```python
from build123d import *

# Parameters (mm, degrees)
F0_R     = 8
F0_R_2   = 16
F1_DEPTH = 19
F0_R_3   = 11
F0_R_4   = 24
F2_DEPTH = 25
F7_DEPTH = 25.001


with BuildPart() as f1:
    # F0 (on Right) → F1 (new body)
    with BuildSketch(Plane.YZ):
        Circle(F0_R)
        Circle(F0_R_2)
        Circle(F0_R, mode=Mode.SUBTRACT)
    extrude(amount=F1_DEPTH)



with BuildPart() as f2:
    # F0 (on Right) → F2 (new body)
    with BuildSketch(Plane.YZ):
        with Locations((0, 140)):
            Circle(F0_R_3)
        with Locations((0, 140)):
            Circle(F0_R_4)
        with Locations((0, 140)):
            Circle(F0_R_3, mode=Mode.SUBTRACT)
    extrude(amount=F2_DEPTH)


with BuildPart() as f1_1:
    add(f1.part)

    add(f2.part)  # F6 merges F2
    # F5 (on plane+point) → F6 section 0
    with BuildSketch(Plane.XY.offset(140)):
        with BuildLine():
            add(Edge.make_bspline(
                [(9, 24), (-1.392305, 24), (3.803848, -12), (9, -48), (14.196152, -12), (19.392305, 24), (9, 24)],
                knots=[0, 0, 0, 2.094395, 2.094395, 4.18879, 4.18879, 6.283185, 6.283185, 6.283185], degree=2, weights=[1, 0.5, 1, 0.5, 1, 0.5, 1]))
        make_face()
    # F3 (on Top) → F6 section 1
    with BuildSketch(Plane.XY):
        with BuildLine():
            add(Edge.make_bspline(
                [(9, 24), (-1.392305, 24), (3.803848, -12), (9, -48), (14.196152, -12), (19.392305, 24), (9, 24)],
                knots=[0, 0, 0, 2.094395, 2.094395, 4.18879, 4.18879, 6.283185, 6.283185, 6.283185], degree=2, weights=[1, 0.5, 1, 0.5, 1, 0.5, 1]))
        make_face()
    loft()

    # F0 (on Right) → F7 (cut, through all)
    with BuildSketch(Plane.YZ):
        with Locations((0, 140)):
            Circle(F0_R_3)
        Circle(F0_R)
    extrude(amount=F7_DEPTH, mode=Mode.SUBTRACT)


solid = f1_1.part
```
Geometry: final body of the model. Coordinates: model frame, mm. A direction names the side the tool comes from. Give positions to 0.01 mm unless a question says otherwise; leave off trailing zeros. Loops run counter-clockwise (first coordinate to the right, second up) from the corner with the lowest first, then second, coordinate; pieces in that order, holes last. Notation, with made-up numbers: (78.5, -1) -> (118.5, -1) arc R17 cw to (118.5, 29) -> close; hole circle Ø6 at (-14, -35.75). An arc over 180 degrees is marked (long way). Use CSV: the item, a comma, the result in double quotes.
(1) Ray query, line 1 along Z through (x, y) = (9.75, 0); line 2 along Z through (x, y) = (16.5, 0); line 3 along Z through (x, y) = (4.5, 3). Return the intervals inside material, ascending. Write a range as [from, to].
From the geometry:
line 1,"[-16, -8], [8, 129], [151, 164]"
line 2,"[-16, -8], [8, 16], [116, 129], [151, 164]"
line 3,"[-15.72, -7.42], [7.42, 129.42], [150.58, 163.81]"
(2) Cut plane A-A (z = 148). Output: boundary loops of the cut face in (x, y), plus the area to 3 significant figures.
From the geometry:
outline,"(0, -22.63) -> (25, -22.63) -> (25, -7.55) -> (0, -7.55) -> close; (0, 7.55) -> (25, 7.55) -> (25, 22.63) -> (0, 22.63) -> close"
area,"754 mm^2"
(3) First-contact query: P1, Ø4, axis at x = 9.5, y = 20, coming from the -Z side; P2, Ø4, axis at x = 21.5, z = 117.5, coming from the +Y side; P3, Ø12, axis at x = 14, y = 16.5, coming from the +Z side. Flat tips, straight axial feed; report the tip coordinate or a pass-through.
From the geometry:
P1,"z = 0"
P2,"y = 12.48"
P3,"z = 161.58"
(4) Cut plane B-B (y = 0). Count the separate pieces of the cut face and the enclosed holes in it, plus the area to 3 significant figures.
From the geometry:
separate pieces,"3"
enclosed holes,"0"
area,"2,150 mm^2"
(5) Access query for faces 1 (the face through (9, 19, 0)), 2 (the face through (19, -7.3, 3.8)), 3 (the face through (9, -19, 0)), 4 (the face through (9.37, -3.47, -15.62)). Directions: +Z, -Z, +X, -X, +Y, -Y. A direction counts if a zero-diameter tool reaches every point of the face in a straight line with its end or side. Return the directions, or none.
From the geometry:
face 1,"-Z, +X, -X, +Y"
face 2,"-Z, +X, +Y, -Y"
face 3,"-Z, +X, -X, -Y"
face 4,"none"
